The figure shows three views and two pictorial views of one solid part (mm, origin at its lowest corner). Answer the questions. A direction names the side the tool comes from. Round coordinates to 2 decimals unless told otherwise and drop trailing zeros. Order: outer loops, then holes, each group sorted by start corner. A loop starts at its lowest first (then second) coordinate and runs counter-clockwise, first axis right, second up. Notation, with made-up numbers: (-39.75, 26.25) -> (-33.75, 26.25) arc R26 cw to (-33.75, 47.25) -> close; hole circle Ø1 at (6.25, 2.5). An arc over 180 degrees is marked (long way). Answer in a Markdown table with one row per item. Add a question column.
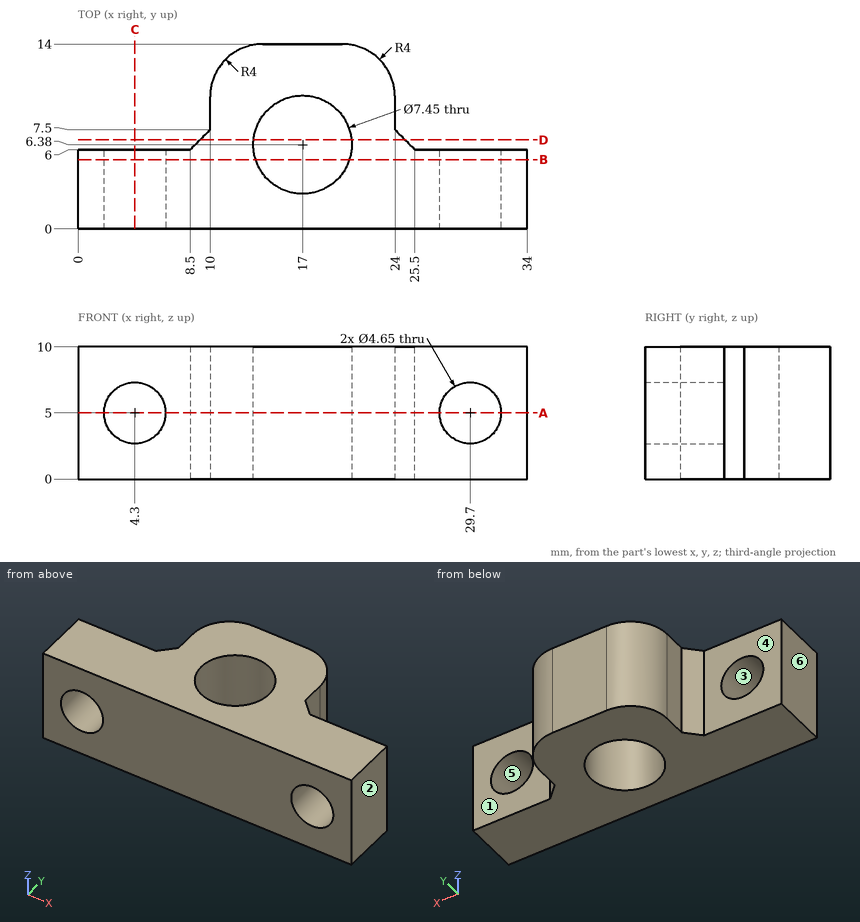
1. The part is cut by section D-D (y = 6.75). Give the vertices of the cut face in (x, z), then the cut area to 3 significant figures.
2. The part is cut by section C-C (x = 4.3). Give the vertices of the cut face in (y, z) (3 decimals).
3. For the marked faces 1 and 2, determine the directions among +Z, -Z, +X, -X, +Y, -Y from which every point of the face is accessible in a straight line to the end or side of a thin tool.
4. Each of these flat-tipped pins is pushed along its axis until it touches: pin 1 (2 mm diameter, centred on x = 12, z = 4.5, fed in from +Y); pin 2 (1 mm diameter, centred on y = 11, z = 4, fed in from -X); pin 3 (5 mm diameter, centred on x = 26, z = 8, fed in from +Y). Where does it stop, or does it pass through?
5. Straight lines are drawn through the part: line 1 along Z through (x, y) = (29.7, 4.05) (3 decimals); line 2 along X through (y, z) = (1.6, 5) (3 decimals); line 3 along Y through (x, z) = (17, 4) (3 decimals). For each, find the intervals that lie inside material, in ascending order.
6. The part is cut by section A-A (z = 5). Give the vertices of the cut face in (x, y) (3 decimals), then the cut area to 3 significant figures.
7. The mould has two halves that part along X. Classify the marked faces 3, 4, 5 and 6: released by +X, released by -X, zero draft, split by the parting line, or undercut.
8. The part is cut by section B-B (y = 5.25). Give the vertices of the cut face in (x, z) (3 decimals), then the cut area to 3 significant figures.
Report:
| question | item | result |
|---|---|---|
| 1 | outline | (9.25, 0) -> (13.29, 0) -> (13.29, 10) -> (9.25, 10) -> close; (20.71, 0) -> (24.75, 0) -> (24.75, 10) -> (20.71, 10) -> close |
| 1 | area | 80.9 mm^2 |
| 2 | outline | (0, 0) -> (6, 0) -> (6, 2.675) -> (0, 2.675) -> close; (0, 7.325) -> (6, 7.325) -> (6, 10) -> (0, 10) -> close |
| 3 | face 1 | +Z, -Z, +X, +Y |
| 3 | face 2 | +Z, -Z, +X, +Y, -Y |
| 4 | pin 1 | stops at y = 13.87 |
| 4 | pin 2 | stops at x = 10.03 |
| 4 | pin 3 | stops at y = 11.94 |
| 5 | line 1 | z = 0 to 2.675, 7.325 to 10 |
| 5 | line 2 | x = 0 to 1.975, 6.625 to 27.375, 32.025 to 34 |
| 5 | line 3 | y = 0 to 2.655, 10.105 to 14 |
| 6 | outline | (0, 0) -> (1.975, 0) -> (1.975, 6) -> (0, 6) -> close; (6.625, 0) -> (27.375, 0) -> (27.375, 6) -> (25.5, 6) -> (24, 7.5) -> (24, 10) arc R4 ccw to (20, 14) -> (14, 14) arc R4 ccw to (10, 10) -> (10, 7.5) -> (8.5, 6) -> (6.625, 6) -> close; (32.025, 0) -> (34, 0) -> (34, 6) -> (32.025, 6) -> close; hole circle Ø7.45 at (17, 6.38) |
| 6 | area | 212 mm^2 |
| 7 | face 3 | undercut |
| 7 | face 4 | zero draft |
| 7 | face 5 | undercut |
| 7 | face 6 | released by -X |
| 8 | outline | (0, 0) -> (13.451, 0) -> (13.451, 10) -> (0, 10) -> close; (20.549, 0) -> (34, 0) -> (34, 10) -> (20.549, 10) -> close; hole circle Ø4.65 at (4.3, 5); hole circle Ø4.65 at (29.7, 5) |
| 8 | area | 235 mm^2 |
